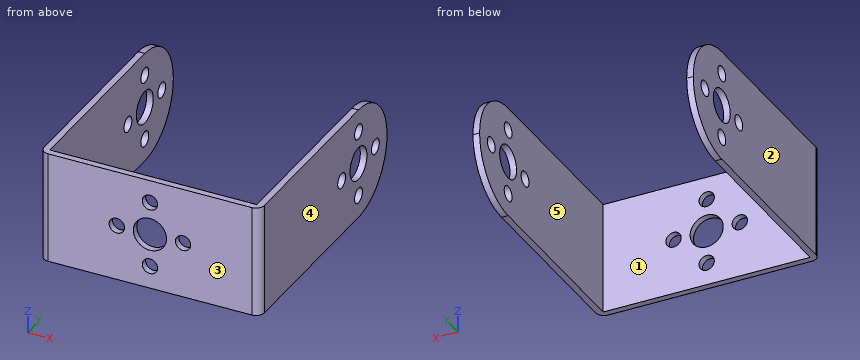
```python
from build123d import *

# Parameters (mm, degrees)
EXTRUDE1_DEPTH           = 27
FILLET2_R                = 13.5
FILLET3_R                = 13.5
FILLET4_R                = 13.5
FILLET5_R                = 13.5
CUT_EXTRUDE1_START       = -53.2
CUT_EXTRUDE1_OUTLINE_R   = 4
CUT_EXTRUDE1_OUTLINE_R_2 = 1.85
CUT_EXTRUDE1_DEPTH       = 53.2
CUT_EXTRUDE2_START       = -1.6
CUT_EXTRUDE2_OUTLINE_R   = 4
CUT_EXTRUDE2_OUTLINE_R_2 = 1.85
CUT_EXTRUDE2_DEPTH       = 1.6
FILLET6_R                = 2
FILLET7_R                = 2


# Read off the part's stored shape, not the designer's step: Cut-Extrude1, Cut-Extrude2
with BuildPart() as part:
    # Sketch1 → Extrude1 (new body)
    with BuildSketch(Plane.XY):
        Polygon((0, 0), (53.2, 0), (53.2, 60.1), (51.6, 60.1), (51.6, 1.6), (1.6, 1.6), (1.6, 60.1), (0, 60.1), align=None)
    extrude(amount=-EXTRUDE1_DEPTH)

    # Fillet2
    fillet2_edges = [part.edges().sort_by_distance(p)[0] for p in [
        (52.4, 60.1, 0),
    ]]
    fillet(fillet2_edges, radius=FILLET2_R)

    # Fillet3
    fillet3_edges = [part.edges().sort_by_distance(p)[0] for p in [
        (52.4, 60.1, -27),
    ]]
    fillet(fillet3_edges, radius=FILLET3_R - 0.0001)  # a hair under: the kernel refuses the full size

    # Fillet4
    fillet4_edges = [part.edges().sort_by_distance(p)[0] for p in [
        (0.8, 60.1, -27),
    ]]
    fillet(fillet4_edges, radius=FILLET4_R)

    # Fillet5
    fillet5_edges = [part.edges().sort_by_distance(p)[0] for p in [
        (0.8, 60.1, 0),
    ]]
    fillet(fillet5_edges, radius=FILLET5_R - 0.0001)  # a hair under: the kernel refuses the full size

    # Cut-Extrude1 outline → Cut-Extrude1 (cut)
    with BuildSketch(Plane(origin=(53.2, 0, 0), x_dir=(0, 0, -1), z_dir=(1, 0, 0)).offset(CUT_EXTRUDE1_START)):
        with Locations((13.5, 46.6)):
            Circle(CUT_EXTRUDE1_OUTLINE_R)
        with Locations((21.5, 46.6)):
            Circle(CUT_EXTRUDE1_OUTLINE_R_2)
        with Locations((5.5, 46.6)):
            Circle(CUT_EXTRUDE1_OUTLINE_R_2)
        with Locations((13.5, 38.6)):
            Circle(CUT_EXTRUDE1_OUTLINE_R_2)
        with Locations((13.5, 54.6)):
            Circle(CUT_EXTRUDE1_OUTLINE_R_2)
    extrude(amount=CUT_EXTRUDE1_DEPTH, mode=Mode.SUBTRACT)

    # Cut-Extrude2 outline → Cut-Extrude2 (cut)
    with BuildSketch(Plane.XZ.offset(CUT_EXTRUDE2_START)):
        with Locations((26.6, -13.5)):
            Circle(CUT_EXTRUDE2_OUTLINE_R)
        with Locations((34.6, -13.5)):
            Circle(CUT_EXTRUDE2_OUTLINE_R_2)
        with Locations((18.6, -13.5)):
            Circle(CUT_EXTRUDE2_OUTLINE_R_2)
        with Locations((26.6, -21.5)):
            Circle(CUT_EXTRUDE2_OUTLINE_R_2)
        with Locations((26.6, -5.5)):
            Circle(CUT_EXTRUDE2_OUTLINE_R_2)
    extrude(amount=CUT_EXTRUDE2_DEPTH, mode=Mode.SUBTRACT)

    # Fillet6
    fillet6_edges = [part.edges().sort_by_distance(p)[0] for p in [
        (53.2, 0, -13.5),
    ]]
    fillet(fillet6_edges, radius=FILLET6_R)

    # Fillet7
    fillet7_edges = [part.edges().sort_by_distance(p)[0] for p in [
        (0, 0, -13.5),
    ]]
    fillet(fillet7_edges, radius=FILLET7_R)


solid = part.part
```
Geometry check sheet. Reference: the model listing, model coordinates, mm. Face numbers are marked on the shaded views. A direction names the side the tool comes from. Round coordinates to 2 decimals unless told otherwise and drop trailing zeros. Write each loop counter-clockwise with the first axis right and the second up, starting at its lowest first coordinate (ties: lowest second). Pieces come first, ordered by that corner, then holes. Notation, with made-up numbers: (-17.5, 71.5) -> (18.5, 71.5) arc R16 ccw to (18.5, 76.5) -> close; hole circle Ø5 at (75.5, 21.5). An arc over 180 degrees is marked (long way). Put each result on its own line as item: value.
1) Cross-section at D-D, the plane y = 54.6. Enter the section's corners in (x, z), plus the area to 3 significant figures.
Recorded:
outline: (0, -24.37) -> (1.6, -24.37) -> (1.6, -15.35) -> (0, -15.35) -> close; (0, -11.65) -> (1.6, -11.65) -> (1.6, -2.63) -> (0, -2.63) -> close; (51.6, -24.37) -> (53.2, -24.37) -> (53.2, -15.35) -> (51.6, -15.35) -> close; (51.6, -11.65) -> (53.2, -11.65) -> (53.2, -2.63) -> (51.6, -2.63) -> close
area: 57.8 mm2
2) Access from +Z, -Z, +X, -X, +Y, -Y to the whole of each face (thin tool, end or side, straight path). Record for the marked faces 4 and 5.
Recorded:
face 4: +Z, -Z, +X, +Y, -Y
face 5: +Z, -Z, +Y
3) Thickness scan on probe 1 along X at (y, z) = (41, -11.5); probe 2 along Z at (x, y) = (34.6, 1.35); probe 3 along Y at (x, z) = (0.5, -13.5). Record the ranges inside material, lowest first. Write a range as from..to.
Recorded:
probe 1: x = 0..1.6, 51.6..53.2
probe 2: z = -27..-15.35, -11.65..0
probe 3: y = 0.68..36.75, 40.45..42.6, 50.6..52.75, 56.45..60.1
4) Cross-section at A-A, the plane y = 21. Enter the section's corners in (x, z).
Recorded:
outline: (0, -27) -> (1.6, -27) -> (1.6, 0) -> (0, 0) -> close; (51.6, -27) -> (53.2, -27) -> (53.2, 0) -> (51.6, 0) -> close
5) Cross-section at B-B, the plane x = 34.6. Enter the section's corners in (y, z).
Recorded:
outline: (0, -27) -> (1.6, -27) -> (1.6, -15.35) -> (0, -15.35) -> close; (0, -11.65) -> (1.6, -11.65) -> (1.6, 0) -> (0, 0) -> close
6) Release check for a two-part mould opening along X. For the marked faces 1, 2 and 3 record: pulls with the +X half, pulls with the -X half, needs draft (parallel to the pull), parting line crosses it, or undercut.
Recorded:
face 1: undercut
face 2: pulls with the -X half
face 3: needs draft
7) Cross-section at C-C, the plane z = -10.5. Enter the section's corners in (x, y).
Recorded:
outline: (0, 2) arc R2 ccw to (2, 0) -> (23.95, 0) -> (23.95, 1.6) -> (1.6, 1.6) -> (1.6, 43.95) -> (0, 43.95) -> close; (0, 49.25) -> (1.6, 49.25) -> (1.6, 59.76) -> (0, 59.76) -> close; (29.25, 0) -> (51.2, 0) arc R2 ccw to (53.2, 2) -> (53.2, 43.95) -> (51.6, 43.95) -> (51.6, 1.6) -> (29.25, 1.6) -> close; (51.6, 49.25) -> (53.2, 49.25) -> (53.2, 59.76) -> (51.6, 59.76) -> close
8) Depth check by flat-ended pin: P1, Ø4.5, axis at x = 26.6, z = -21.5, coming from the +Y side; P2, Ø3.5, axis at x = 34.6, z = -13.5, coming from the -Y side. Enter the tip coordinate at first touch or a pass-through.
Recorded:
P1: stops at y = 1.6
P2: passes through
